```python
from build123d import *

# Parameters (mm, degrees)
BOSS_EXTRUDE1_DEPTH = 3.5
FILLET1_R           = 3
FILLET2_R           = 3
FILLET3_R           = 1
CUT_EXTRUDE1_DEPTH  = 4.5


with BuildPart() as part:
    # Sketch1 → Boss-Extrude1 (new, symmetric)
    with BuildSketch(Plane(origin=(0, 0, 0), x_dir=(1, 0, 0), z_dir=(0, 1, 0))):
        Polygon((5, 0), (-5, 0), (-5, 8), (-12, 8), (-12, 10), (12, 10), (12, 8), (5, 8), align=None)
    extrude(amount=BOSS_EXTRUDE1_DEPTH, both=True)

    # Fillet1
    fillet1_edges = [part.edges().sort_by_distance(p)[0] for p in [
        (12, 3.5, -9),
        (-12, 3.5, -9),
        (-12, -3.5, -9),
        (12, -3.5, -9),
    ]]
    fillet(fillet1_edges, radius=FILLET1_R)

    # Fillet2
    fillet2_edges = [part.edges().sort_by_distance(p)[0] for p in [
        (-5, 0, -8),
        (5, 0, -8),
    ]]
    fillet(fillet2_edges, radius=FILLET2_R)

    # Fillet3
    fillet3_edges = [part.edges().sort_by_distance(p)[0] for p in [
        (5, 3.5, -2.5),
        (5, -3.5, -2.5),
        (5.878679656, -3.5, -7.121320344),
        (11.121320344, -2.621320344, -8),
        (11.121320344, 2.621320344, -8),
        (-5, -3.5, -2.5),
        (-5.878679656, -3.5, -7.121320344),
        (-11.121320344, -2.621320344, -8),
        (-11.121320344, 2.621320344, -8),
        (-5, 3.5, -2.5),
        (5.878679656, 3.5, -7.121320344),
        (-5.878679656, 3.5, -7.121320344),
        (0, 3.5, -10),
        (-11.121320344, 2.621320344, -10),
        (-11.121320344, -2.621320344, -10),
        (0, -3.5, -10),
        (11.121320344, -2.621320344, -10),
        (11.121320344, 2.621320344, -10),
        (12, 0, -8),
        (-12, 0, -8),
        (12, 0, -10),
        (-12, 0, -10),
        (8.5, -3.5, -8),
        (8.5, 3.5, -8),
        (-8.5, -3.5, -8),
        (-8.5, 3.5, -8),
    ]]
    fillet(fillet3_edges, radius=FILLET3_R - 0.0001)  # a hair under: the kernel refuses the full size

    # Sketch3 → Cut-Extrude1 (cut)
    with BuildSketch(Plane.XY):
        Polygon((2.45, 0), (0, 2.45), (-2.45, 0), (0, -2.45), align=None)
    extrude(amount=-CUT_EXTRUDE1_DEPTH, mode=Mode.SUBTRACT)


solid = part.part
```
Could you check a few things on this model? Use its own coordinates, in mm. A direction names the side the tool comes from. Give positions to 0.01 mm unless a question says otherwise; leave off trailing zeros. Loops run counter-clockwise (first coordinate to the right, second up) from the corner with the lowest first, then second, coordinate; pieces in that order, holes last. Notation, with made-up numbers: (84, 12) -> (112, 12) arc R27 cw to (112, 29) -> close; hole circle Ø6 at (-19.5, 24). An arc over 180 degrees is marked (long way). Put each result on its own line as item: value.
(1) I'm going to push flat-ended pins straight in: pin 1 Ø4 at (y, z) = (0.5, -1.5) entering from -X; pin 2 Ø4 at (x, y) = (-9, 1.5) entering from +Z; pin 3 Ø1.5 at (x, y) = (-9, -0.5) entering from +Z; pin 4 Ø2.5 at (x, y) = (-1, -0.5) entering from +Z. Where does each tip first touch, or does it pass through?
Computed:
pin 1: x = -5
pin 2: z = -7.83
pin 3: z = -8
pin 4: z = 0
(2) Please list where these lines run through material, in increasing order: probe 1 along Z at (x, y) = (-10, 2); probe 2 along X at (y, z) = (-1, -1.75); probe 3 along X at (y, z) = (1.25, -5). Write a range as [from, to].
Computed:
probe 1: [-10, -8]
probe 2: [-5, -1.45], [1.45, 5]
probe 3: [-5, 5]
(3) Imagine slicing it at B-B on x = 0.5. Write out the boundary of the cut face in (y, z), plus the area to 3 significant figures.
Computed:
outline: (-3.5, -9) arc R1 ccw to (-2.5, -10) -> (2.5, -10) arc R1 ccw to (3.5, -9) -> (3.5, 0) -> (1.95, 0) -> (1.95, -4.5) -> (-1.95, -4.5) -> (-1.95, 0) -> (-3.5, 0) -> close
area: 52.0 mm^2
(4) Imagine slicing it at A-A on z = -1.75. Write out the boundary of the cut face in (x, y).
Computed:
outline: (-5, -2.5) arc R1 ccw to (-4, -3.5) -> (4, -3.5) arc R1 ccw to (5, -2.5) -> (5, 2.5) arc R1 ccw to (4, 3.5) -> (-4, 3.5) arc R1 ccw to (-5, 2.5) -> close; hole (-2.45, 0) -> (0, -2.45) -> (2.45, 0) -> (0, 2.45) -> close
(5) For faces 1 (the face through (-8.507, -3.199, -8.285)), 2 (the face through (4.699, 3.215, -2.465)), 3 (the face through (10, 0, -8)), 4 (the face through (-9, 0, -8)), 5 (the face through (-8.493, 3.199, -8.285)), which set-ups out of +Z, -Z, +X, -X, +Y, -Y let a thin tool reach every point of the face, with its end or its side?
Computed:
face 1: +Z, -X, -Y
face 2: +Z, +X, +Y
face 3: +Z, +X, +Y, -Y
face 4: +Z, -X, +Y, -Y
face 5: +Z, -X, +Y
